Work out the finished part from the listing and answer in its coordinate system (mm). A direction names the side the tool comes from. Give positions to 0.01 mm unless a question says otherwise; leave off trailing zeros. Order: outer loops, then holes, each group sorted by start corner. A loop starts at its lowest first (then second) coordinate and runs counter-clockwise, first axis right, second up. Notation, with made-up numbers: (37.5, 9) -> (70.5, 9) arc R31 ccw to (70.5, 43) -> close; hole circle Ø10 at (-6, -4.75). An arc over 180 degrees is marked (long way). Answer as CSV lines item,"result". Start each with the question number.
1. Find the intervals of material crossed by L1, parallel to X at y = 16, z = 9; L2, parallel to Y at x = -17, z = 3.5; L3, parallel to Z at x = 6.5, y = -6.5, in increasing order.
2. A cutting plane is placed at A-A (z = 9.25). Give the vertices of the cut face in (x, y), then the cut area to 3 significant figures.
3. For faces 4 (the flat face through (-17, 17, 4)), 5 (the flat face through (-14, -17.5, 2.7)), 6 (the flat face through (21, 17, 6)), 7 (the flat face through (-19, 19, 7)), determine the directions among +Z, -Z, +X, -X, +Y, -Y from which every point of the face is accessible in a straight line to the end or side of a thin tool.
4. A cutting plane is placed at C-C (x = -16). Give the vertices of the cut face in (y, z), then the cut area to 3 significant figures.
5. For a pull along X with two mould halves and no side action, classify faces 1 (the flat face through (-20, -1, 6)), 2 (the flat face through (-41, 1, 1)), 3 (the flat face through (-32, 17, 1)) as released by +X, released by -X, zero draft, split by the parting line, or undercut.
6. Flat-ended cylindrical pins translate along their axes: pin 1 (1.6 mm diameter, centred on x = 5.5, z = 0.5, fed in from +Y); pin 2 (1.6 mm diameter, centred on x = -21, y = -7.5, fed in from +Z); pin 3 (4 mm diameter, centred on x = 19.5, z = 8, fed in from +Y); pin 4 (5 mm diameter, centred on x = 13, y = -10.5, fed in from +Z). Find the tip coordinate at first contact, or state that the pin passes through.
from build123d import *

# Parameters (mm, degrees)
F1_DEPTH  = 2
F2_W      = 3
F2_H      = 17
F3_DEPTH  = 10
F4_W      = 10
F4_H      = 2
F5_DEPTH  = 2
F6_SIZE   = 1.99999
F2_H_2    = 10
F2_H_3    = 7
F7_DEPTH  = 5
F8_DEPTH  = 7
F9_W      = 17
F9_H      = 2
F10_DEPTH = 2
F11_SIZE  = 1.99999
F14_DEPTH = 2
F15_SIZE  = 1.99999
F17_DEPTH = 3
F18_R     = 0.5
F19_DEPTH = 3.001
F21_DEPTH = 1.9


# Not quite as in the source:
# - a fillet or chamfer is up to 0.001 mm smaller than in the source, because OpenCascade refuses the exact size
# - a feature names something its author has since deleted; it is built from what else it names


with BuildPart() as f1:
    # F0 (on Top) → F1 (new body)
    with BuildSketch(Plane.XY):
        with BuildLine():
            Line((-14, 17), (-15, 17))
            Line((-15, 17), (-20, 17))
            Line((-20, 17), (-20, -15))
            Line((-20, -15), (-20, -17))
            Line((-20, -17), (-15, -17))
            Line((-15, -17), (-14, -17))
            Line((-14, -17), (-14, -15))
            ThreePointArc((-14, -15), (-11.6568542495, -9.3431457505), (-6, -7))
            Line((-6, -7), (12, -7))
            ThreePointArc((12, -7), (17.6568542495, -9.3431457505), (20, -15))
            Line((20, -15), (20, 15))
            ThreePointArc((20, 15), (17.6568542495, 9.3431457505), (12, 7))
            Line((12, 7), (-6, 7))
            ThreePointArc((-6, 7), (-11.6568542495, 9.3431457505), (-14, 15))
            Line((-14, 15), (-14, 17))
        make_face()
        Polygon((-20, -15), (-20, 17), (-23, 17), (-23, -17), (-20, -17), align=None)
        with BuildLine():
            Line((22, 17), (20, 17))
            Line((20, 17), (20, 15))
            Line((20, 15), (20, -15))
            Line((20, -15), (20, -17))
            Line((20, -17), (22, -17))
            ThreePointArc((22, -17), (22.7071067812, -16.7071067812), (23, -16))
            Line((23, -16), (23, 16))
            ThreePointArc((23, 16), (22.7071067812, 16.7071067812), (22, 17))
        make_face()
    extrude(amount=F1_DEPTH)

    # F2 (on face) → F3 (join)
    with BuildSketch(Plane.XY.offset(2)):
        with BuildLine():
            Line((20, -7), (20, -15))
            Line((20, -15), (20, -17))
            Line((20, -17), (22, -17))
            ThreePointArc((22, -17), (22.7071067812, -16.7071067812), (23, -16))
            Line((23, -16), (23, -7))
            Line((23, -7), (20, -7))
        make_face()
        with BuildLine():
            Line((20, 15), (20, 7))
            Line((20, 7), (23, 7))
            Line((23, 7), (23, 16))
            ThreePointArc((23, 16), (22.7071067812, 16.7071067812), (22, 17))
            Line((22, 17), (20, 17))
            Line((20, 17), (20, 15))
        make_face()
        with Locations((-21.5, 8.5)):
            Rectangle(F2_W, F2_H)
    extrude(amount=F3_DEPTH)

    # F4 (on face) → F5 (join)
    with BuildSketch(Plane(origin=(20, 0, 0), x_dir=(0, -1, 0), z_dir=(-1, 0, 0))):
        with Locations((-12, 11)):
            Rectangle(F4_W, F4_H)
        with Locations((12, 11)):
            Rectangle(F4_W, F4_H)
    extrude(amount=F5_DEPTH)

    # F6 (size 2 in the source; OpenCascade refuses exactly that, so slightly less here)
    f6_edges = [f1.edges().sort_by_distance(p)[0] for p in [
        (18, 12, 10),
        (18, -12, 10),
    ]]
    chamfer(f6_edges, length=F6_SIZE)

    # F2 (on face) → F7 (join)
    with BuildSketch(Plane.XY.offset(2)):
        with Locations((-21.5, -12)):
            Rectangle(F2_W, F2_H_2)
        with Locations((-21.5, -3.5)):
            Rectangle(F2_W, F2_H_3)
    extrude(amount=F7_DEPTH)

    # F0 (on Top) → F8 (join)
    with BuildSketch(Plane.XY):
        with BuildLine():
            Line((-15, -17), (-20, -17))
            Line((-20, -17), (-23, -17))
            Line((-23, -17), (-23, -19))
            ThreePointArc((-23, -19), (-22.7071067812, -19.7071067812), (-22, -20))
            Line((-22, -20), (-15, -20))
            ThreePointArc((-15, -20), (-14.2928932188, -19.7071067812), (-14, -19))
            Line((-14, -19), (-14, -18))
            Line((-14, -18), (-14, -17))
            Line((-14, -17), (-15, -17))
        make_face()
        with BuildLine():
            Line((-20, 17), (-15, 17))
            Line((-15, 17), (-14, 17))
            Line((-14, 17), (-14, 18))
            Line((-14, 18), (-14, 19))
            ThreePointArc((-14, 19), (-14.2928932188, 19.7071067812), (-15, 20))
            Line((-15, 20), (-22, 20))
            ThreePointArc((-22, 20), (-22.7071067812, 19.7071067812), (-23, 19))
            Line((-23, 19), (-23, 17))
            Line((-23, 17), (-20, 17))
        make_face()
    extrude(amount=F8_DEPTH)

    # F9 (on face) → F10 (join)
    with BuildSketch(Plane.YZ.offset(-20)):
        with Locations((8.5, 11)):
            Rectangle(F9_W, F9_H)
    extrude(amount=F10_DEPTH)

    # F11 (size 2 in the source; OpenCascade refuses exactly that, so slightly less here)
    f11_edges = [f1.edges().sort_by_distance(p)[0] for p in [
        (-18, 8.5, 10),
    ]]
    chamfer(f11_edges, length=F11_SIZE)

    # F13 (on face) → F14 (join)
    with BuildSketch(Plane.YZ.offset(-20)):
        Polygon((-9.5, 7), (-11, 7), (-11, 5), (-8, 5), (-8, 7), align=None)
        Polygon((-1, 5), (-1, 7), (-2.5, 7), (-4, 7), (-4, 5), align=None)
    extrude(amount=F14_DEPTH)

    # F15 (size 2 in the source; OpenCascade refuses exactly that, so slightly less here)
    f15_edges = [f1.edges().sort_by_distance(p)[0] for p in [
        (-18, -9.5, 5),
        (-18, -2.5, 5),
    ]]
    chamfer(f15_edges, length=F15_SIZE)

    # F16 (on face) → F17 (cut)
    with BuildSketch(Plane.XY.offset(7)):
        Polygon((-23, 0), (-23, -1), (-23, -4), (-21, -4), (-21, -1), (-20, -1), (-20, 0), align=None)
        Polygon((-21, -4), (-23, -4), (-23, -5), (-20, -5), (-20, -4), align=None)
        Polygon((-21, -8), (-23, -8), (-23, -11), (-23, -12), (-21, -12), (-20, -12), (-20, -11), (-21, -11), align=None)
        Polygon((-21, -7), (-23, -7), (-23, -8), (-21, -8), (-20, -8), (-20, -7), align=None)
    extrude(amount=-F17_DEPTH, mode=Mode.SUBTRACT)

    # F18 (on face) → F19 (cut, through all)
    with BuildSketch(Plane.YZ.offset(-20)):
        with Locations((-9.5, 4)):
            Circle(F18_R)
        with Locations((-2.5, 4)):
            Circle(F18_R)
    extrude(amount=-F19_DEPTH, mode=Mode.SUBTRACT)

    # F20 (on Top) → F21 (join)
    with BuildSketch(Plane.XY):
        with BuildLine():
            Line((-23, -19), (-23, -17))
            Line((-23, -17), (-23, 17))
            Line((-23, 17), (-23, 19))
            Line((-23, 19), (-23, 20))
            Line((-23, 20), (-25.5, 20))
            ThreePointArc((-25.5, 20), (-26.5606601718, 19.5606601718), (-27, 18.5))
            ThreePointArc((-27, 18.5), (-27.4393398282, 17.4393398282), (-28.5, 17))
            Line((-28.5, 17), (-35.5, 17))
            ThreePointArc((-35.5, 17), (-36.5606601718, 17.4393398282), (-37, 18.5))
            ThreePointArc((-37, 18.5), (-37.4393398282, 19.5606601718), (-38.5, 20))
            Line((-38.5, 20), (-39, 20))
            ThreePointArc((-39, 20), (-40.4142135624, 19.4142135624), (-41, 18))
            Line((-41, 18), (-41, 16))
            Line((-41, 16), (-41, -16))
            ThreePointArc((-41, -16), (-39.8284271247, -18.8284271247), (-37, -20))
            Line((-37, -20), (-23, -20))
            Line((-23, -20), (-23, -19))
        make_face()
        with BuildLine():
            Line((-23, 20), (-23, 19))
            ThreePointArc((-23, 19), (-22.7071067812, 19.7071067812), (-22, 20))
            Line((-22, 20), (-23, 20))
        make_face()
        with BuildLine():
            ThreePointArc((-22, -20), (-22.7071067812, -19.7071067812), (-23, -19))
            Line((-23, -19), (-23, -20))
            Line((-23, -20), (-22, -20))
        make_face()
    extrude(amount=F21_DEPTH)


solid = f1.part
Answer sheet:
1,L1,"x = -23 to -20, 20 to 23"
1,L2,"y = -20 to -17, 17 to 20"
1,L3,"z = 0 to 2"
2,outline,"(-23, 0) -> (-20, 0) -> (-20, 17) -> (-23, 17) -> close; (20, -17) -> (22, -17) arc R1 ccw to (23, -16) -> (23, -7) -> (20, -7) -> close; (20, 7) -> (23, 7) -> (23, 16) arc R1 ccw to (22, 17) -> (20, 17) -> close"
2,area,"111 mm^2"
3,face 4,"none"
3,face 5,"+Z, -Z, -Y"
3,face 6,"+Z, -Z, +X, +Y"
3,face 7,"+Z, +X, -X, +Y"
4,outline,"(-20, 0) -> (20, 0) -> (20, 7) -> (17, 7) -> (17, 2) -> (-17, 2) -> (-17, 7) -> (-20, 7) -> close"
4,area,"110 mm^2"
5,face 1,"zero draft"
5,face 2,"released by -X"
5,face 3,"undercut"
6,pin 1,"stops at y = 7"
6,pin 2,"stops at z = 7"
6,pin 3,"stops at y = 17"
6,pin 4,"passes through"
